from build123d import *

# Parameters (mm, degrees)
BOSS_EXTRUDE1_DEPTH = 32.5
SKETCH2_R           = 2.75
CUT_EXTRUDE1_DEPTH  = 2
CUT_EXTRUDE2_DEPTH  = 2
SKETCH4_W           = 25
SKETCH4_H           = 13
BOSS_EXTRUDE2_DEPTH = 2
CUT_EXTRUDE3_REACH  = 55.742
CUT_EXTRUDE4_REACH  = 55.742
SKETCH7_W           = 7
SKETCH7_H           = 13


with BuildPart() as part:
    # Sketch1 → Boss-Extrude1 (new body)
    with BuildSketch(Plane(origin=(0, 0, 0), x_dir=(0, 1, 0), z_dir=(0, 0, 1))):
        Polygon((0, 0), (0, -15), (23, -15), (23, -17), (-2, -17), (-2, 0), align=None)
    extrude(amount=BOSS_EXTRUDE1_DEPTH)

    # Sketch2 → Cut-Extrude1 (cut)
    with BuildSketch(Plane.XZ.offset(2)):
        with Locations((8, 25.25)):
            Circle(SKETCH2_R)
        with Locations((8, 7.25)):
            Circle(SKETCH2_R)
    extrude(amount=-CUT_EXTRUDE1_DEPTH, mode=Mode.SUBTRACT)

    # Sketch3 → Cut-Extrude2 (cut)
    with BuildSketch(Plane.YZ.offset(17)):
        Polygon((23, 22.5), (0, 0), (23, 0), align=None)
    extrude(amount=-CUT_EXTRUDE2_DEPTH, mode=Mode.SUBTRACT)

    # Sketch4 → Boss-Extrude2 (add)
    with BuildSketch(Plane.YZ.offset(17)):
        with Locations((10.5, 39)):
            Rectangle(SKETCH4_W, SKETCH4_H)
    extrude(amount=-BOSS_EXTRUDE2_DEPTH)

    # Sketch5 → Cut-Extrude3 (cut, up to next)
    with BuildSketch(Plane.YZ.offset(17), mode=Mode.PRIVATE) as cut_extrude3_sk1:
        with BuildLine():
            Line((8.925, 41.025), (19.575, 41.025))
            ThreePointArc((19.575, 41.025), (20.5, 40.1), (19.575, 39.175))
            Line((19.575, 39.175), (8.925, 39.175))
            ThreePointArc((8.925, 39.175), (8, 40.1), (8.925, 41.025))
        make_face()
    cut_extrude3_tool1 = extrude(cut_extrude3_sk1.sketch, amount=-CUT_EXTRUDE3_REACH, mode=Mode.PRIVATE) & part.part
    # Sketch5 → Cut-Extrude3 (cut, up to next)
    with BuildSketch(Plane.YZ.offset(17), mode=Mode.PRIVATE) as cut_extrude3_sk2:
        with BuildLine():
            Line((8.925, 32.175), (19.575, 32.175))
            ThreePointArc((19.575, 32.175), (20.5, 31.25), (19.575, 30.325))
            Line((19.575, 30.325), (8.925, 30.325))
            ThreePointArc((8.925, 30.325), (8, 31.25), (8.925, 32.175))
        make_face()
    cut_extrude3_tool2 = extrude(cut_extrude3_sk2.sketch, amount=-CUT_EXTRUDE3_REACH, mode=Mode.PRIVATE) & part.part
    add(cut_extrude3_tool1.solids().sort_by_distance((17, 14.25, 40.1))[0], mode=Mode.SUBTRACT)
    add(cut_extrude3_tool2.solids().sort_by_distance((17, 14.25, 31.25))[0], mode=Mode.SUBTRACT)

    # Sketch7 → Cut-Extrude4 (cut, up to next)
    with BuildSketch(Plane.YZ.offset(17), mode=Mode.PRIVATE) as cut_extrude4_sk1:
        with Locations((1.5, 39)):
            Rectangle(SKETCH7_W, SKETCH7_H)
    cut_extrude4_tool1 = extrude(cut_extrude4_sk1.sketch, amount=-CUT_EXTRUDE4_REACH, mode=Mode.PRIVATE) & part.part
    add(cut_extrude4_tool1.solids().sort_by_distance((17, 1.5, 39))[0], mode=Mode.SUBTRACT)


solid = part.part
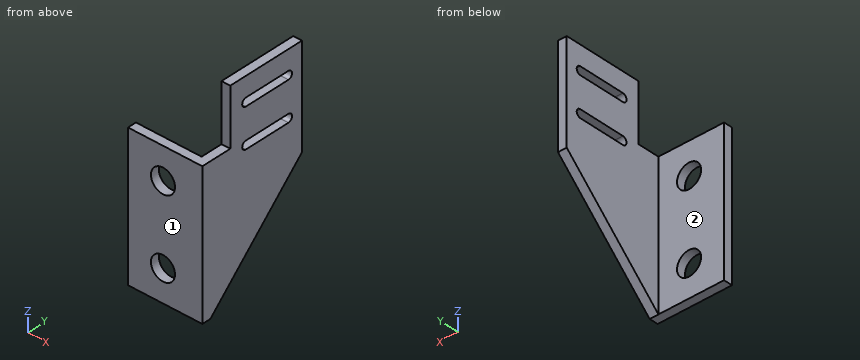
Read the model definition and answer for the solid it produces. Units are mm, in the model's axes. Face numbers are marked on the shaded views. A direction names the side the tool comes from. Coordinates: 2 decimals unless noted, no trailing zeros. Order: outer loops, then holes, each group sorted by start corner. A loop starts at its lowest first (then second) coordinate and runs counter-clockwise, first axis right, second up. Notation, with made-up numbers: (63.25, -35) - (83.25, -35) arc R34 cw to (83.25, 0) - close; hole circle Ø3 at (47.25, 60). An arc over 180 degrees is marked (long way). Use one line per item in the form item = value.
(1) Given pin 1 Ø1.5 at (x, y) = (14.5, 14.5) entering from -Z; pin 2 Ø2 at (y, z) = (11.5, 19.5) entering from -X; pin 3 Ø4.5 at (x, z) = (8, 7.25) entering from +Y; pin 4 Ø2 at (x, z) = (15.5, 38.5) entering from -Y, each flat-ended and moving along its own axis, determine where each tip first touches the part or whether it passes through.
Computed values:
pin_1 = 13.64
pin_2 = 15
pin_3 = through
pin_4 = 5
(2) Which of the six approach directions +Z, -Z, +X, -X, +Y, -Y give full straight-line access (tool end or side, diameter ignored) to the marked faces 1 and 2?
Computed values:
face_1 = +Z, -Z, +X, -X, -Y
face_2 = +Z, -Z, -X, +Y
(3) Section D-D, the plane x = 8 is taken. Give the vertices of the cut face in (y, z), then the cut area to 3 significant figures.
Computed values:
outline = (-2, 0) - (0, 0) - (0, 4.5) - (-2, 4.5) - close; (-2, 10) - (0, 10) - (0, 22.5) - (-2, 22.5) - close; (-2, 28) - (0, 28) - (0, 32.5) - (-2, 32.5) - close
area = 43.0 mm²
(4) Section B-B, the plane x = 15.5 is taken. Give the vertices of the cut face in (y, z) (3 decimals).
Computed values:
outline = (-2, 0) - (0, 0) - (23, 22.5) - (23, 45.5) - (5, 45.5) - (5, 32.5) - (-2, 32.5) - close; hole (8.925, 30.325) - (19.575, 30.325) arc R0.925 ccw to (19.575, 32.175) - (8.925, 32.175) arc R0.925 ccw to start; hole (8.925, 39.175) - (19.575, 39.175) arc R0.925 ccw to (19.575, 41.025) - (8.925, 41.025) arc R0.925 ccw to start
(5) Straight lines are drawn through the part: L1, parallel to Z at x = 8, y = -1.15; L2, parallel to X at y = 5.5, z = 18.5; L3, parallel to Y at x = 4, z = 25. For each, find the intervals that lie inside material, in ascending order.
Computed values:
L1 = 0 to 4.5, 10 to 22.5, 28 to 32.5
L2 = 15 to 17
L3 = -2 to 0
(6) Section C-C, the plane y = 18.75 is taken. Give the vertices of the cut face in (x, z) (3 decimals), then the cut area to 3 significant figures.
Computed values:
outline = (15, 18.342) - (17, 18.342) - (17, 30.325) - (15, 30.325) - close; (15, 32.175) - (17, 32.175) - (17, 39.175) - (15, 39.175) - close; (15, 41.025) - (17, 41.025) - (17, 45.5) - (15, 45.5) - close
area = 46.9 mm²
(7) Section A-A, the plane z = 25.25 is taken. Give the vertices of the cut face in (x, y), then the cut area to 3 significant figures.
Computed values:
outline = (0, -2) - (5.25, -2) - (5.25, 0) - (0, 0) - close; (10.75, -2) - (17, -2) - (17, 23) - (15, 23) - (15, 0) - (10.75, 0) - close
area = 69.0 mm²
